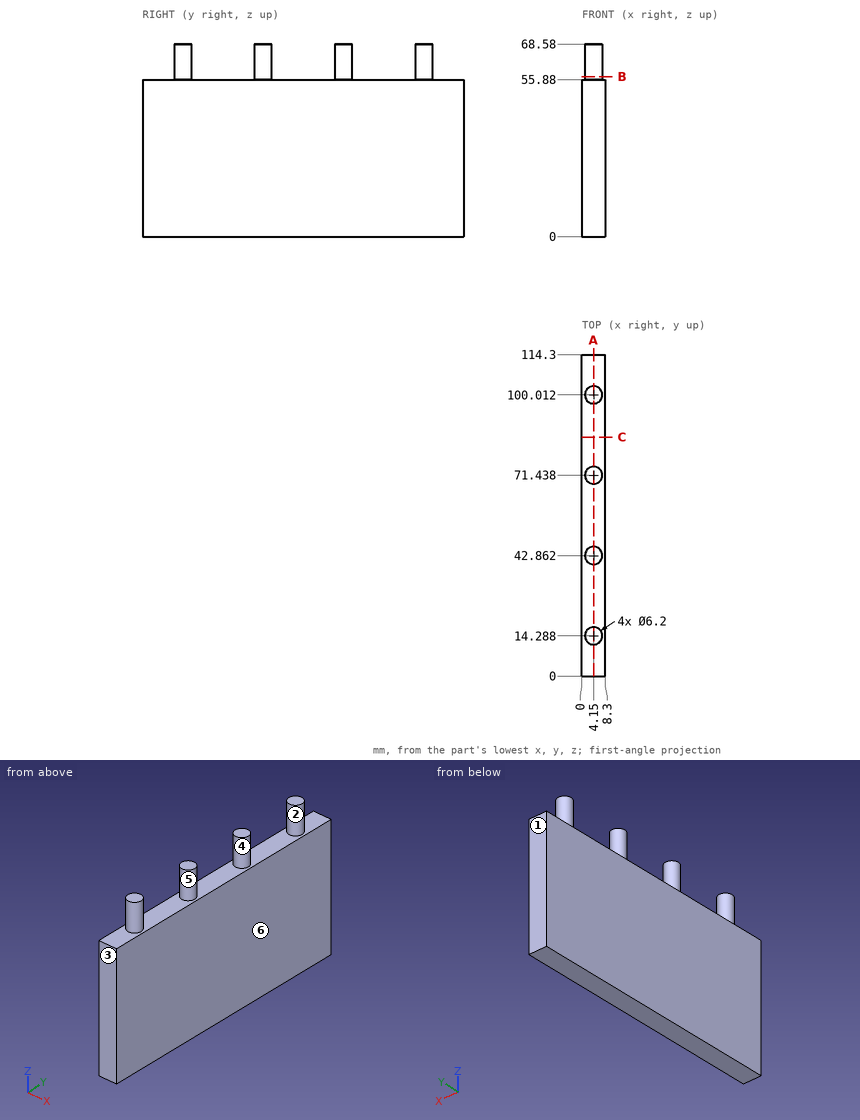
Print and shaded views of the part. All mm, measured from the part's lowest x, y and z. A direction names the side the tool comes from. Coordinates: 2 decimals unless noted, no trailing zeros. Write each loop counter-clockwise with the first axis right and the second up, starting at its lowest first coordinate (ties: lowest second). Pieces come first, ordered by that corner, then holes. Notation, with made-up numbers: (31.5, 2) - (74.5, 2) arc R22 ccw to (74.5, 34) - close; hole circle Ø11 at (38.5, 73). An arc over 180 degrees is marked (long way). One line per question, with ' | ' between items. Start each with the question number.
Q1. Drill centre lines: line 1 (Y direction, x = 4, z = 56.5); line 2 (Y direction, x = 2.5, z = 66.5) (1 decimal); line 3 (Z direction, x = 7, y = 35). Where is each one in solid material? Low to high. Write a range as [from, to].
Q2. Pull direction Y, two halves, no side cores. Call the marked faces 3, 4, 5 and 6: pulls with the +Y half, pulls with the -Y half, needs draft (parallel to the pull), parting line crosses it, or undercut.
Q3. 3-axis set-ups, long thin cutter, end or side, ignore diameter. For the marked faces 1 and 2: which of +Z, -Z, +X, -X, +Y, -Y reach the whole face in a straight line?
Q4. Cut at C-C, the plane y = 85. List the corners of the cut face in (x, z), then the cut area to 3 significant figures.
Q5. Cut at B-B, the plane z = 57. List the corners of the cut face in (x, y), then the cut area to 3 significant figures.
Q6. Pin check, flat tips, straight feed: pin 1 (5 mm diameter, centred on y = 12, z = 59, fed in from +X); pin 2 (1.5 mm diameter, centred on y = 17.5, z = 60.5, fed in from -X) (1 decimal); pin 3 (4 mm diameter, centred on x = 2.5, y = 94, fed in from +Z). Stop position of each tip, or through.
Q7. Cut at A-A, the plane x = 4.15. List the corners of the cut face in (y, z), then the cut area to 3 significant figures.
Answer below:
1) line 1: [11.19, 17.38], [39.77, 45.96], [68.34, 74.53], [96.92, 103.11] | line 2: [11.7, 16.9], [40.2, 45.5], [68.8, 74.1], [97.4, 102.6] | line 3: [0, 55.88]
2) face 3: pulls with the -Y half | face 4: undercut | face 5: undercut | face 6: needs draft
3) face 1: +Z, -Z, +X, -X, +Y | face 2: +Z
4) outline: (0, 0) - (8.3, 0) - (8.3, 55.88) - (0, 55.88) - close | area: 464 mm^2
5) outline: circle Ø6.2 at (4.15, 14.29); circle Ø6.2 at (4.15, 42.86); circle Ø6.2 at (4.15, 71.44); circle Ø6.2 at (4.15, 100.01) | area: 121 mm^2
6) pin 1: x = 7.25 | pin 2: x = 2.3 | pin 3: z = 55.88
7) outline: (0, 0) - (114.3, 0) - (114.3, 55.88) - (103.11, 55.88) - (103.11, 68.58) - (96.91, 68.58) - (96.91, 55.88) - (74.54, 55.88) - (74.54, 68.58) - (68.34, 68.58) - (68.34, 55.88) - (45.96, 55.88) - (45.96, 68.58) - (39.76, 68.58) - (39.76, 55.88) - (17.39, 55.88) - (17.39, 68.58) - (11.19, 68.58) - (11.19, 55.88) - (0, 55.88) - close | area: 6,700 mm^2
